```python
from build123d import *

# Parameters (mm, degrees)
SKETCH1_R           = 4
BOSS_EXTRUDE1_DEPTH = 6.5


with BuildPart() as part:
    # Sketch1 → Boss-Extrude1 (new body)
    with BuildSketch(Plane.XY):
        Polygon((0, -7.505553499), (6.5, -3.75277675), (6.5, 3.75277675), (0, 7.505553499), (-6.5, 3.75277675), (-6.5, -3.75277675), align=None)
        with Locations(Location((0, 0, 0), (0, 0, 180))):
            Circle(SKETCH1_R, mode=Mode.SUBTRACT)
    extrude(amount=BOSS_EXTRUDE1_DEPTH)

    # Sketch2 → Cut-Revolve1 (revolve, cut)
    with BuildSketch(Plane(origin=(0, 0, 0), x_dir=(0, 0, -1), z_dir=(1, 0, 0)), mode=Mode.PRIVATE) as cut_revolve1_sk:
        Polygon((-6.5, 7.505553499), (-6.5, 6.5), (-5.958333333, 7.505553499), align=None)
        Polygon((-0.541666667, 7.505553499), (0, 7.505553499), (0, 6.5), align=None)
        Polygon((-6.5, 4), (-5.85, 4), (-6.5, 4.65), align=None)
        Polygon((0, 4), (-0.65, 4), (0, 4.65), align=None)
    revolve(cut_revolve1_sk.sketch.rotate(Axis((0, 0, 0), (0, 0, 1)), 90), axis=Axis((0, 0, 0), (0, 0, 1)), mode=Mode.SUBTRACT)


solid = part.part
```
Input: part model. Units: mm. Frame: model coordinates. Coordinates: 2 decimals unless noted, no trailing zeros. Write each loop counter-clockwise with the first axis right and the second up, starting at its lowest first coordinate (ties: lowest second). Pieces come first, ordered by that corner, then holes.
1) Pin query (flat end, axial travel): pin 1 Ø6.5 at (x, y) = (0, 0) entering from -Z; pin 2 Ø3 at (x, y) = (-3, 5.5) entering from -Z; pin 3 Ø3 at (x, z) = (-5, 2.5) entering from +Y. Return the tip coordinate at first contact, or that it passes through.
2) Mould query, pull axis X, two halves, no side actions, for faces 1 (the conical face through (-0.02, -6.74, 0.13)), 2 (the flat face through (6.5, 0, 3)), 3 (the conical face through (-5.849, -3.358, 6.368)). Classes: pulls with the +X half, pulls with the -X half, needs draft (parallel to the pull), parting line crosses it, or undercut.
3) Section A-A on z = 2.25. Output: boundary loops of the cut face in (x, y), and give its area (3 significant figures).
4) Material intervals for line 1 along Y through (x, z) = (-1.75, 0.75); line 2 along Y through (x, z) = (0.25, 6); line 3 along X through (y, z) = (2, 6.25), sorted ascending.
Check result:
1. pin 1: passes through
1. pin 2: stops at z = 0
1. pin 3: stops at y = 5.48
2. face 1: parting line crosses it
2. face 2: pulls with the +X half
2. face 3: pulls with the -X half
3. outline: (-6.5, -3.75) - (0, -7.51) - (6.5, -3.75) - (6.5, 3.75) - (0, 7.51) - (-6.5, 3.75) - close; hole circle Ø8 at (0, 0)
3. area: 96.1 mm2
4. line 1: y = -6.5 to -3.6, 3.6 to 6.5
4. line 2: y = -7.36 to -4.14, 4.14 to 7.36
4. line 3: x = -6.5 to -3.92, 3.92 to 6.5
